CAD build for the part. Positions are in the model's coordinates, mm. A direction names the side the tool comes from. Round coordinates to 2 decimals unless told otherwise and drop trailing zeros. Loops run counter-clockwise (first coordinate to the right, second up) from the corner with the lowest first, then second, coordinate; pieces in that order, holes last. Notation, with made-up numbers: M 15,-25.75 L 43,-25.75 A27 cw 43,2.25 Z; hole C -38.75,86.5 d7. An arc over 180 degrees is marked long. Use a Markdown table: item, result. Add a question column.
(1) Band-saw the part on B-B, the plane z = 5.5. Write the cut outline in (x, y), and give its area (3 significant figures).
(2) Two-plate mould, pull along Z, no slides. Class faces 1 (the face through (22, 1, 25)), 2 (the face through (22, 2, 0)), 3 (the face through (14, 4, 1)): released by +Z, released by -Z, zero draft, split by the parting line, or undercut.
(3) Flat gauge pins, fed straight in: P1, Ø0.8, axis at x = 16.5, y = 3.5, coming from the +Z side; P2, Ø6, axis at x = 24, z = 20.5, coming from the +Y side; P3, Ø6, axis at x = 16, z = 8.5, coming from the +Y side. Where does each tip first touch, or does it go through?
(4) Which spindle directions (+Z, -Z, +X, -X, +Y, -Y) get a long thin tool onto all of the face, cutting with end or side? Do faces 4 (the face through (17.25, 4, 4)), 5 (the face through (15.75, 4, 4)), 6 (the face through (18.549, 3.116, 0.74)), 7 (the face through (16, 4, 6.5)). Say none if no direction does.
(5) Wall check: L1, parallel to Y at x = 12, z = 28; L2, parallel to Y at x = 39, z = 40.5; L3, parallel to Z at x = 17.5, y = 4.25. Give the ranges that are in metal, low to high.
(6) Band-saw the part on A-A, the plane x = 22. Write the cut outline in (y, z), and give its area (3 significant figures).
(7) Band-saw the part on C-C, the plane x = 30. Write the cut outline in (y, z), and give its area (4 significant figures).
(8) Band-saw the part on D-D, the plane z = 21. Write the cut outline in (x, y).
from build123d import *

# Parameters (mm, degrees)
CROQUIS1_W              = 45
CROQUIS1_H              = 50.5
SALIENTE_EXTRUIR1_DEPTH = 2
CROQUIS10_W             = 29
CROQUIS10_H             = 34.5
CORTAR_EXTRUIR5_DEPTH   = 1
CORTAR_EXTRUIR6_DEPTH   = 1
CROQUIS6_W              = 17
CROQUIS6_H              = 4.5
SALIENTE_EXTRUIR5_DEPTH = 1.5
CORTAR_EXTRUIR4_REACH   = 52.5
CROQUIS9_W              = 1.5
CROQUIS9_H              = 3.5
SALIENTE_EXTRUIR6_DEPTH = 5


with BuildPart() as part:
    # Croquis1 → Saliente-Extruir1 (new body)
    with BuildSketch(Plane(origin=(0, 0, 0), x_dir=(1, 0, 0), z_dir=(0, 1, 0))):
        with Locations((22.5, -25.25)):
            Rectangle(CROQUIS1_W, CROQUIS1_H)
    extrude(amount=SALIENTE_EXTRUIR1_DEPTH)

    # Croquis10 → Cortar-Extruir5 (cut)
    with BuildSketch(Plane(origin=(0, 2, 0), x_dir=(1, 0, 0), z_dir=(0, 1, 0))):
        with Locations((22.5, -25.25)):
            Rectangle(CROQUIS10_W, CROQUIS10_H)
    extrude(amount=-CORTAR_EXTRUIR5_DEPTH, mode=Mode.SUBTRACT)

    # Croquis11 → Cortar-Extruir6 (cut)
    with BuildSketch(Plane.XZ):
        Polygon((45, 0), (45, 50.5), (0, 50.5), (0, 0), (1, 0), (1, 49.5), (44, 49.5), (44, 0), align=None)
    extrude(amount=-CORTAR_EXTRUIR6_DEPTH, mode=Mode.SUBTRACT)

    # Croquis6 → Saliente-Extruir5 (add)
    with BuildSketch(Plane(origin=(0, 0, 0), x_dir=(-1, 0, 0), z_dir=(0, 0, -1))):
        with Locations((-22.5, 4.25)):
            Rectangle(CROQUIS6_W, CROQUIS6_H)
    extrude(amount=-SALIENTE_EXTRUIR5_DEPTH)

    # Croquis8 → Cortar-Extruir4 (cut, up to next)
    with BuildSketch(Plane(origin=(0, 0, 0), x_dir=(-1, 0, 0), z_dir=(0, 0, -1)), mode=Mode.PRIVATE) as cortar_extruir4_sk1:
        with BuildLine():
            Line((-19.16109127, 5.94246212), (-18.55753788, 5.33890873))
            ThreePointArc((-18.55753788, 5.33890873), (-18.329926491, 4.998264213), (-18.25, 4.596446609))
            Line((-18.25, 4.596446609), (-18.25, 3.85))
            ThreePointArc((-18.25, 3.85), (-18.55753788, 3.10753788), (-19.3, 2.8))
            Line((-19.3, 2.8), (-25.7, 2.8))
            ThreePointArc((-25.7, 2.8), (-26.44246212, 3.10753788), (-26.75, 3.85))
            Line((-26.75, 3.85), (-26.75, 4.596446609))
            ThreePointArc((-26.75, 4.596446609), (-26.670073509, 4.998264213), (-26.44246212, 5.33890873))
            Line((-26.44246212, 5.33890873), (-25.83890873, 5.94246212))
            ThreePointArc((-25.83890873, 5.94246212), (-25.498264213, 6.170073509), (-25.096446609, 6.25))
            Line((-25.096446609, 6.25), (-19.903553391, 6.25))
            ThreePointArc((-19.903553391, 6.25), (-19.501735787, 6.170073509), (-19.16109127, 5.94246212))
        make_face()
    cortar_extruir4_tool1 = extrude(cortar_extruir4_sk1.sketch, amount=-CORTAR_EXTRUIR4_REACH, mode=Mode.PRIVATE) & part.part
    add(cortar_extruir4_tool1.solids().sort_by_distance((22.5, 4.475322, 0))[0], mode=Mode.SUBTRACT)

    # Croquis9 → Saliente-Extruir6 (add)
    with BuildSketch(Plane.XY.offset(1.5)):
        with Locations((28.5, 3.75)):
            Rectangle(CROQUIS9_W, CROQUIS9_H)
        with Locations((16.5, 3.75)):
            Rectangle(CROQUIS9_W, CROQUIS9_H)
    extrude(amount=SALIENTE_EXTRUIR6_DEPTH)


solid = part.part
Return value:
| question | item | result |
|---|---|---|
| 1 | outline | M 0,1 L 1,1 L 1,0 L 44,0 L 44,1 L 45,1 L 45,2 L 29.25,2 L 29.25,5.5 L 27.75,5.5 L 27.75,2 L 17.25,2 L 17.25,5.5 L 15.75,5.5 L 15.75,2 L 0,2 Z |
| 1 | area | 98.5 mm^2 |
| 2 | face 1 | undercut |
| 2 | face 2 | released by -Z |
| 2 | face 3 | zero draft |
| 3 | P1 | z = 6.5 |
| 3 | P2 | y = 1 |
| 3 | P3 | y = 5.5 |
| 4 | face 4 | +Z, +Y |
| 4 | face 5 | +Z, -X, +Y |
| 4 | face 6 | +Z, -Z |
| 4 | face 7 | +Z, +X, -X, +Y |
| 5 | L1 | 0 to 1 |
| 5 | L2 | 0 to 2 |
| 5 | L3 | 0 to 1.5 |
| 6 | outline | M 0,0 L 2.8,0 L 2.8,1.5 L 2,1.5 L 2,8 L 1,8 L 1,42.5 L 2,42.5 L 2,50.5 L 1,50.5 L 1,49.5 L 0,49.5 Z; M 6.25,0 L 6.5,0 L 6.5,1.5 L 6.25,1.5 Z |
| 6 | area | 67.1 mm^2 |
| 7 | outline | M 0,0 L 6.5,0 L 6.5,1.5 L 2,1.5 L 2,8 L 1,8 L 1,42.5 L 2,42.5 L 2,50.5 L 1,50.5 L 1,49.5 L 0,49.5 Z |
| 7 | area | 72.25 mm^2 |
| 8 | outline | M 0,1 L 1,1 L 1,0 L 44,0 L 44,1 L 45,1 L 45,2 L 37,2 L 37,1 L 8,1 L 8,2 L 0,2 Z |
